from build123d import *

# Parameters (mm, degrees)
F0_R      = 500
F1_DEPTH  = 100
F2_R      = 10
F3_DEPTH  = 100.001
F4_W      = 20
F4_H      = 15
F4_W_2    = 5
F4_W_3    = 10
F4_H_2    = 110
F5_DEPTH  = 50
F6_W      = 20
F6_H      = 20
F6_W_2    = 10
F6_H_2    = 100
F7_DEPTH  = 50
F8_W      = 20
F8_H      = 110
F9_DEPTH  = 50
F10_W     = 20
F10_H     = 10
F10_W_2   = 5
F10_H_2   = 120
F11_DEPTH = 50
F12_W     = 20
F12_H     = 10
F12_W_2   = 5
F12_H_2   = 120
F13_DEPTH = 50
F14_R     = 10
F15_DEPTH = 10
F16_R     = 500
F16_R_2   = 490
F17_DEPTH = 20
F19_DEPTH = 50
F21_DEPTH = 50


with BuildPart() as f1:
    # F0 (on Top) → F1 (new body)
    with BuildSketch(Plane.XY):
        Circle(F0_R)
    extrude(amount=F1_DEPTH)

    # F2 (on face) → F3 (cut, through all)
    with BuildSketch(Plane.XY.offset(100)):
        Circle(F2_R)
    extrude(amount=-F3_DEPTH, mode=Mode.SUBTRACT)

    # F4 (on face) → F5 (cut)
    with BuildSketch(Plane.XY.offset(100)):
        Polygon((-60, 470), (-80, 470), (-50, 400), (-40, 423.3333333333), align=None)
        Polygon((-40, 423.3333333333), (-50, 400), (-40, 376.6666666667), (-30, 400), align=None)
        Polygon((-40, 376.6666666667), (-50, 400), (-80, 330), (-60, 330), align=None)
        Polygon((-30, 400), (-40, 376.6666666667), (-20, 330), (0, 330), align=None)
        Polygon((-20, 470), (-40, 423.3333333333), (-30, 400), (0, 470), align=None)
        with Locations((20, 462.5)):
            Rectangle(F4_W, F4_H)
        with Locations((7.5, 462.5)):
            Rectangle(F4_W_2, F4_H)
        with Locations((35, 462.5)):
            Rectangle(F4_W_3, F4_H)
        with Locations((20, 400)):
            Rectangle(F4_W, F4_H_2)
        with Locations((50, 462.5)):
            Rectangle(F4_W, F4_H)
        with Locations((20, 337.5)):
            Rectangle(F4_W, F4_H)
        with Locations((7.5, 337.5)):
            Rectangle(F4_W_2, F4_H)
        with Locations((35, 337.5)):
            Rectangle(F4_W_3, F4_H)
        with Locations((50, 400)):
            Rectangle(F4_W, F4_H_2)
        with Locations((62.5, 462.5)):
            Rectangle(F4_W_2, F4_H)
        with Locations((50, 337.5)):
            Rectangle(F4_W, F4_H)
        with Locations((62.5, 337.5)):
            Rectangle(F4_W_2, F4_H)
    extrude(amount=-F5_DEPTH, mode=Mode.SUBTRACT)

    # F6 (on face) → F7 (cut)
    with BuildSketch(Plane.XY.offset(100)):
        with Locations((400, 60)):
            Rectangle(F6_W, F6_H)
        with Locations((385, 60)):
            Rectangle(F6_W_2, F6_H)
        with Locations((415, 60)):
            Rectangle(F6_W_2, F6_H)
        with Locations((370, 60)):
            Rectangle(F6_W, F6_H)
        with Locations((430, 60)):
            Rectangle(F6_W, F6_H)
        with Locations((400, -60)):
            Rectangle(F6_W, F6_H)
        with Locations((385, -60)):
            Rectangle(F6_W_2, F6_H)
        with Locations((370, 0)):
            Rectangle(F6_W, F6_H_2)
        with Locations((355, 60)):
            Rectangle(F6_W_2, F6_H)
        with Locations((415, -60)):
            Rectangle(F6_W_2, F6_H)
        with Locations((430, 0)):
            Rectangle(F6_W, F6_H_2)
        with Locations((445, 60)):
            Rectangle(F6_W_2, F6_H)
        with Locations((370, -60)):
            Rectangle(F6_W, F6_H)
        with Locations((430, -60)):
            Rectangle(F6_W, F6_H)
        with Locations((355, -60)):
            Rectangle(F6_W_2, F6_H)
        with Locations((445, -60)):
            Rectangle(F6_W_2, F6_H)
    extrude(amount=-F7_DEPTH, mode=Mode.SUBTRACT)

    # F8 (on face) → F9 (cut)
    with BuildSketch(Plane.XY.offset(100)):
        with Locations((400, 0)):
            Rectangle(F8_W, F8_H)
    extrude(amount=-F9_DEPTH, mode=Mode.SUBTRACT)

    # F10 (on face) → F11 (cut)
    with BuildSketch(Plane.XY.offset(100)):
        Polygon((-40, -330), (-60, -330), (-30, -470), (-20, -423.3333333333), align=None)
        Polygon((-20, -423.3333333333), (-30, -470), (-10, -470), align=None)
        Polygon((0, -330), (-20, -423.3333333333), (-10, -470), (20, -330), align=None)
        with Locations((40, -335)):
            Rectangle(F10_W, F10_H)
        with Locations((27.5, -335)):
            Rectangle(F10_W_2, F10_H)
        with Locations((52.5, -335)):
            Rectangle(F10_W_2, F10_H)
        with Locations((40, -400)):
            Rectangle(F10_W, F10_H_2)
        with Locations((40, -465)):
            Rectangle(F10_W, F10_H)
        with Locations((27.5, -465)):
            Rectangle(F10_W_2, F10_H)
        with Locations((52.5, -465)):
            Rectangle(F10_W_2, F10_H)
    extrude(amount=-F11_DEPTH, mode=Mode.SUBTRACT)

    # F12 (on face) → F13 (cut)
    with BuildSketch(Plane.XY.offset(100)):
        Polygon((-400, 70), (-420, 70), (-390, 0), (-380, 23.3333333333), align=None)
        Polygon((-380, 23.3333333333), (-390, 0), (-380, -23.3333333333), (-370, 0), align=None)
        Polygon((-380, -23.3333333333), (-390, 0), (-420, -70), (-400, -70), align=None)
        Polygon((-370, 0), (-380, -23.3333333333), (-360, -70), (-340, -70), align=None)
        Polygon((-360, 70), (-380, 23.3333333333), (-370, 0), (-340, 70), align=None)
        with Locations((-440, 65)):
            Rectangle(F12_W, F12_H)
        with Locations((-452.5, 65)):
            Rectangle(F12_W_2, F12_H)
        with Locations((-427.5, 65)):
            Rectangle(F12_W_2, F12_H)
        with Locations((-440, 0)):
            Rectangle(F12_W, F12_H_2)
        with Locations((-440, -65)):
            Rectangle(F12_W, F12_H)
        with Locations((-452.5, -65)):
            Rectangle(F12_W_2, F12_H)
        with Locations((-427.5, -65)):
            Rectangle(F12_W_2, F12_H)
    extrude(amount=-F13_DEPTH, mode=Mode.SUBTRACT)

    # F14 (on face) → F15 (cut)
    with BuildSketch(Plane(origin=(0, 0, 0), x_dir=(1, 0, 0), z_dir=(0, 0, -1))):
        with Locations((-230, 0)):
            Circle(F14_R)
    extrude(amount=-F15_DEPTH, mode=Mode.SUBTRACT)

    # F16 (on face) → F17 (join)
    with BuildSketch(Plane.XY.offset(100)):
        Circle(F16_R)
        Circle(F16_R_2, mode=Mode.SUBTRACT)
    extrude(amount=F17_DEPTH)

    # F18 (on face) → F19 (cut)
    with BuildSketch(Plane.XY.offset(100)):
        Polygon((87.867965, 212.132035), (0, 300), (-87.867965, 212.132035), align=None)
        Polygon((87.867965, 212.132035), (-87.867965, 212.132035), (-212.132035, 87.867965), (-212.132035, -87.867965), (-87.867965, -212.132035), (87.867965, -212.132035), (212.132035, -87.867965), (212.132035, 87.867965), align=None)
        Polygon((-212.132035, 87.867965), (-87.867965, 212.132035), (-212.132035, 212.132035), align=None)
        Polygon((212.132035, 212.132035), (87.867965, 212.132035), (212.132035, 87.867965), align=None)
        Polygon((-212.132035, -87.867965), (-212.132035, 87.867965), (-300, 0), align=None)
        Polygon((300, 0), (212.132035, 87.867965), (212.132035, -87.867965), align=None)
        Polygon((-87.867965, -212.132035), (-212.132035, -87.867965), (-212.132035, -212.132035), align=None)
        Polygon((212.132035, -212.132035), (212.132035, -87.867965), (87.867965, -212.132035), align=None)
        Polygon((87.867965, -212.132035), (-87.867965, -212.132035), (0, -300), align=None)
    extrude(amount=-F19_DEPTH, mode=Mode.SUBTRACT)

    # F20 (on face) → F21 (join)
    with BuildSketch(Plane.XY.offset(50)):
        Polygon((58.578645, 141.421355), (0, 200), (-58.578645, 141.421355), align=None)
        Polygon((58.578645, 141.421355), (-58.578645, 141.421355), (-141.421355, 58.578645), (-141.421355, -58.578645), (-58.578645, -141.421355), (58.578645, -141.421355), (141.421355, -58.578645), (141.421355, 58.578645), align=None)
        Polygon((-141.421355, 58.578645), (-58.578645, 141.421355), (-141.421355, 141.421355), align=None)
        Polygon((141.421355, 141.421355), (58.578645, 141.421355), (141.421355, 58.578645), align=None)
        Polygon((-141.421355, -58.578645), (-141.421355, 58.578645), (-200, 0), align=None)
        Polygon((200, 0), (141.421355, 58.578645), (141.421355, -58.578645), align=None)
        Polygon((-58.578645, -141.421355), (-141.421355, -58.578645), (-141.421355, -141.421355), align=None)
        Polygon((141.421355, -141.421355), (141.421355, -58.578645), (58.578645, -141.421355), align=None)
        Polygon((58.578645, -141.421355), (-58.578645, -141.421355), (0, -200), align=None)
    extrude(amount=F21_DEPTH)


solid = f1.part
Geometry: final body of the model. Coordinates: model frame, mm. Give positions to 0.01 mm unless a question says otherwise; leave off trailing zeros. Order: outer loops, then holes, each group sorted by start corner. A loop starts at its lowest first (then second) coordinate and runs counter-clockwise, first axis right, second up. Notation, with made-up numbers: (63.5, 41) -> (79.5, 41) arc R8 cw to (79.5, 56) -> close; hole circle Ø7 at (32, 9). An arc over 180 degrees is marked (long way). Put each result on its own line as item: value.
Q1. Material intervals for L1, parallel to Y at x = 0, z = 114; L2, parallel to X at y = -74.5, z = 84; L3, parallel to Y at x = 0, z = 39, sorted ascending.
Here are the results:
L1: y = -500 to -490, 490 to 500
L2: x = -494.42 to -225.5, -141.42 to 141.42, 225.5 to 494.42
L3: y = -500 to -10, 10 to 500
Q2. Section C-C, the plane y = 259.5. Return loops of the section in (x, z).
Here are the results:
outline: (-427.39, 0) -> (427.39, 0) -> (427.39, 120) -> (415.64, 120) -> (415.64, 100) -> (40.5, 100) -> (40.5, 50) -> (-40.5, 50) -> (-40.5, 100) -> (-415.64, 100) -> (-415.64, 120) -> (-427.39, 120) -> close
Q3. Section B-B, the plane y = -368. Return loops of the section in (x, z).
Here are the results:
outline: (-338.49, 0) -> (338.49, 0) -> (338.49, 120) -> (323.54, 120) -> (323.54, 100) -> (50, 100) -> (50, 50) -> (30, 50) -> (30, 100) -> (11.86, 100) -> (11.86, 50) -> (-8.14, 50) -> (-8.14, 100) -> (-31.86, 100) -> (-31.86, 50) -> (-51.86, 50) -> (-51.86, 100) -> (-323.54, 100) -> (-323.54, 120) -> (-338.49, 120) -> close
Q4. Draft query along Y for faces 1 (the face through (368, -331, 120)), 2 (the face through (-30, -170, 75)). Return one class per face: released by +Y, released by -Y, zero draft, split by the parting line, or undercut.
Here are the results:
face 1: zero draft
face 2: undercut
Q5. Pin query (flat end, axial travel): pin 1 (3 mm diameter, centred on y = -65.5, z = 85.5, fed in from +X); pin 2 (6 mm diameter, centred on x = -72.5, z = 78.5, fed in from -Y); pin 3 (3 mm diameter, centred on x = 357.5, z = 69, fed in from -Y). Return the tip coordinate at first contact, or that it passes through.
Here are the results:
pin 1: stops at x = 495.89
pin 2: stops at y = -495.15
pin 3: stops at y = -351.09
Q6. Section A-A, the plane z = 74. Count the separate pieces of the cut face and the enclosed holes in it, then the cut area to 3 significant figures.
Here are the results:
separate pieces: 5
enclosed holes: 8
area: 631,000 mm^2
